Autodesk Inventor part; units mm, degrees
ref_plane "YZ Plane" through (0, 0, 0) normal (1, 0, 0) x (0, 1, 0)
ref_plane "XZ Plane" through (0, 0, 0) normal (0, 1, 0) x (-1, 0, 0)
ref_plane "XY Plane" through (0, 0, 0) normal (0, 0, 1) x (1, 0, 0)
sketch "Sketch1" plane through (0, 0, 0) normal (0, 0, 1) x (1, 0, 0)
  point P0 (0, 0)
sketch "Sketch2" plane through (0, 0, 0) normal (0, 0, 1) x (1, 0, 0)
  line L0 (-9.1353, 0) -> (-5.9, 0)
  arc A0 (-1, 9.0804) -> (-9.1353, 0) centre (0, 0) ccw
  line L1 (-1, 9.0804) -> (-1, 5.8146)
  arc A1 (1, 5.8146) -> (-1, 5.8146) centre (0, 0) ccw
  line L2 (1, 5.8146) -> (1, 9.0804)
  arc A2 (9.1353, 0) -> (1, 9.0804) centre (0, 0) ccw
  line L3 (5.9, 0) -> (9.1353, 0)
  arc A3 (4.9167, -3.2613) -> (5.9, 0) centre (0, 0) ccw
  line L4 (4.9167, -3.2613) -> (5.7, -9.8727)
  arc A4 (5.7, -9.8727) -> (-5.7, -9.8727) centre (0, 0) ccw
  line L5 (-4.9167, -3.2613) -> (-5.7, -9.8727)
  arc A5 (-5.9, 0) -> (-4.9167, -3.2613) centre (0, 0) ccw
  line L6 (-16.1, 0) -> (16.1, 0)
  line L7 (0, -14.2512) -> (0, 15.7919)
  dimension "d1" = 0
  dimension "d3" = 5.9
  dimension "d5" = 11.4
  dimension "d7" = 0
  dimension "d9" = 9.1353
  dimension "d11" = 1
  dimension "d13" = 1
  dimension "d15" = 5.7
  dimension "d17" = 5.7
  dimension "d19" = 9.8333
extrude "Extrusion1" add sketch "Sketch2" along normal blind 1.1 contours L6 A4 L7 A1 L1 A0 | L0 A5 L5 A4 L6 | A4 L6 A2 L2 A1 L7 | L3 L6 A4 L4 A3
fillet "Fillet1" radius 1.4182 4 edges at (-9.1353, 0, 0.55) (-1, 9.0804, 0.55) (1, 9.0804, 0.55) (9.1353, 0, 0.55)
chamfer "Chamfer1" distance 1.14 distance2 1.7333 1 edges at (-5.7, -9.8727, 0.55) measured on face at (9.3111, 6.5775, 0.3667)
chamfer "Chamfer2" distance 1.7333 distance2 1.14 1 edges at (5.7, -9.8727, 0.55) measured on face at (5.4389, -7.6689, 0.3667)
equation "\"d23\" = 0.05 * Diam3"
equation "\"d24\" = 0.222222 * Diam3 - 0.222222 * sd"
equation "\"d25\" = 0.222222 * Diam3 - 0.222222 * sd"
equation "\"d26\" = 0.05 * Diam3"
equation "\"d3\" = 0.5 * Diam"
equation "\"d5\" = 0.5 * Diam3"
equation "\"d9\" = 0.294118 * Diam3 + 0.205882 * Diam"
equation "\"d11\" = 0.0909091 * Diam3 - 0.0909091 * Diam"
equation "\"d13\" = 0.0909091 * Diam3 - 0.0909091 * Diam"
equation "\"d15\" = 0.25 * Diam3"
equation "\"d17\" = 0.25 * Diam3"
equation "\"d19\" = 0.833333 * Diam"
equation "\"d20\" = ParT"
equation "\"d22\" = 0.181818 * Diam3 - 0.181818 * sd"
equation "\"Diam3\" = 22.8"
equation "\"ParT\" = 1.1"
equation "\"Diam\" = 11.8"
equation "\"sd\" = 15"
equation "\"TEMPLATE\" = 1.2345"
properties part number "ANSI B27.7M - 3CMI-15" material "Steel, Mild"
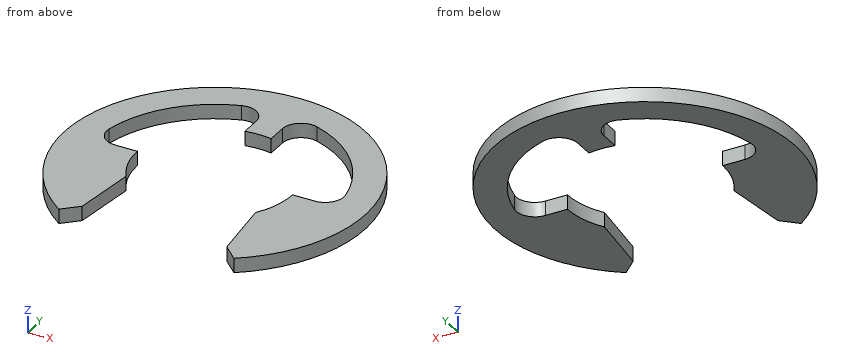
Source: CAD feature listing. Evaluate the final solid. Frame: model axes, mm. Coordinates: 2 decimals unless noted, no trailing zeros. Loops run counter-clockwise (first coordinate to the right, second up) from the corner with the lowest first, then second, coordinate; pieces in that order, holes last. Notation, with made-up numbers: (68, 58.25) -> (93, 58.25) arc R30 ccw to (93, 81.25) -> close; hole circle Ø3 at (-2.5, -30). An arc over 180 degrees is marked (long way). One line per item, written item: value. Start each with the question number.
Q1. Section query C-C, the plane x = 0. Return the cut outline in (y, z), and give its area (3 significant figures).
Q2. Section query A-A, the plane y = -4. Return the cut outline in (x, z).
Q3. Line query: line 1 along X through (y, z) = (6.5, 1); line 2 along X through (y, z) = (-5.75, 0.1); line 3 along Y through (x, z) = (-6.5, 0.8). Output: solid intervals per line, ascending.
Q4. Section query B-B, the plane z = 0.7. Return the cut outline in (x, y), and give its area (3 significant figures).
Q5. Section query D-D, the plane y = -7.25. Return the cut outline in (x, z), and give its area (3 significant figures).
Results:
1. outline: (5.9, 0) -> (11.4, 0) -> (11.4, 1.1) -> (5.9, 1.1) -> close
1. area: 6.05 mm^2
2. outline: (-10.68, 0) -> (-5, 0) -> (-5, 1.1) -> (-10.68, 1.1) -> close; (5, 0) -> (10.68, 0) -> (10.68, 1.1) -> (5, 1.1) -> close
3. line 1: -9.37 to -6.42, -1 to 1, 6.42 to 9.37
3. line 2: -9.84 to -5.21, 5.21 to 9.84
3. line 3: -9.1 to 0, 6.42 to 9.37
4. outline: (-8.98, 1.68) arc R9.14 cw to (-2.86, 8.68) arc R1.42 cw to (-1, 7.33) -> (-1, 5.81) arc R5.9 cw to (1, 5.81) -> (1, 7.33) arc R1.42 cw to (2.86, 8.68) arc R9.14 cw to (8.98, 1.68) arc R1.42 cw to (7.59, 0) -> (5.9, 0) arc R5.9 cw to (4.92, -3.26) -> (5.5, -8.15) -> (6.66, -9.25) arc R11.4 ccw (long way) to (-6.66, -9.25) -> (-5.5, -8.15) -> (-4.92, -3.26) arc R5.9 cw to (-5.9, 0) -> (-7.59, 0) arc R1.42 cw to start
4. area: 166 mm^2
5. outline: (-8.8, 0) -> (-5.39, 0) -> (-5.39, 1.1) -> (-8.8, 1.1) -> close; (5.39, 0) -> (8.8, 0) -> (8.8, 1.1) -> (5.39, 1.1) -> close
5. area: 7.50 mm^2
